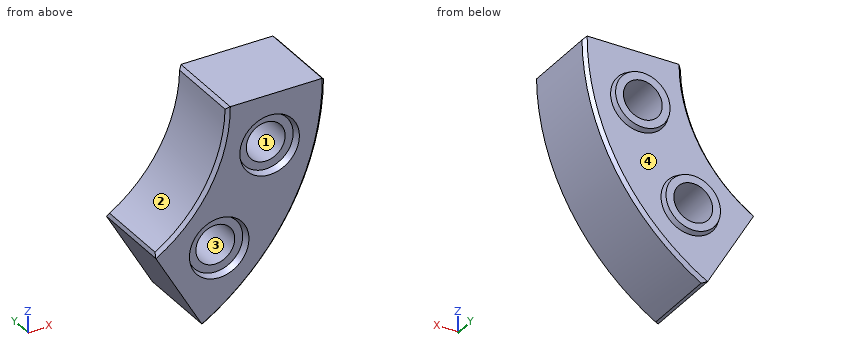
```python
from build123d import *
from OCP.BRepFilletAPI import BRepFilletAPI_MakeChamfer

# Parameters (mm, degrees)
SKETCH1_R           = 30
BOSS_EXTRUDE1_DEPTH = 127
BOSS_EXTRUDE2_START = 8
SKETCH2_R           = 45
SKETCH2_R_2         = 30
BOSS_EXTRUDE2_DEPTH = 8
CHAMFER1_SIZE       = 2.911761874
CHAMFER1_SIZE_2     = 8
CUT_EXTRUDE1_START  = -10
SKETCH3_R           = 46
SKETCH3_R_2         = 30
CUT_EXTRUDE1_DEPTH  = 10
CHAMFER2_SIZE       = 3.639702343
CHAMFER2_SIZE_2     = 10


# Some blends are built 0.0001 mm under size
with BuildPart() as part:
    # Sketch1 → Boss-Extrude1 (new body)
    with BuildSketch(Plane(origin=(0, 0, 0), x_dir=(1, 0, 0), z_dir=(0, 1, 0))):
        with BuildLine():
            Line((225, 0), (377, 0))
            ThreePointArc((377, 0), (326.491577227, 188.5), (188.5, 326.491577227))
            Line((188.5, 326.491577227), (112.5, 194.855715852))
            ThreePointArc((112.5, 194.855715852), (194.855715851, 112.5), (225, 0))
        make_face()
        with Locations(Location((212.839141137, 212.839141137, 0), (0, 0, 270))):
            Circle(SKETCH1_R, mode=Mode.SUBTRACT)
        with Locations(Location((290.743673713, 77.904532576, 0), (0, 0, 270))):
            Circle(SKETCH1_R, mode=Mode.SUBTRACT)
    extrude(amount=-BOSS_EXTRUDE1_DEPTH)

    # Sketch2 → Boss-Extrude2 (add)
    # profile 1 of 2: a face of its own
    with BuildSketch(Plane(origin=(0, 0, 0), x_dir=(1, 0, 0), z_dir=(0, 1, 0)).offset(BOSS_EXTRUDE2_START)):
        with Locations(Location((212.839141137, 212.839141137, 0), (0, 0, 270))):
            Circle(SKETCH2_R)
        with Locations(Location((212.839141137, 212.839141137, 0), (0, 0, 270))):
            Circle(SKETCH2_R_2, mode=Mode.SUBTRACT)
    # profile 2 of 2: a face of its own
    with BuildSketch(Plane(origin=(0, 0, 0), x_dir=(1, 0, 0), z_dir=(0, 1, 0)).offset(BOSS_EXTRUDE2_START)):
        with Locations(Location((290.743673713, 77.904532576, 0), (0, 0, 270))):
            Circle(SKETCH2_R)
        with Locations(Location((290.743673713, 77.904532576, 0), (0, 0, 270))):
            Circle(SKETCH2_R_2, mode=Mode.SUBTRACT)
    extrude(amount=-BOSS_EXTRUDE2_DEPTH)

    # Chamfer1
    chamfer1_edges_1 = [part.edges().sort_by_distance(p)[0] for p in [
        (212.839141137, 8, -257.839141137),
    ]]
    chamfer1_side_1 = [part.faces().sort_by_distance(p)[0] for p in [
        (212.839141137, 8, -257.7809059),
    ]]
    chamfer1_edges_2 = [part.edges().sort_by_distance(p)[0] for p in [
        (290.743673713, 8, -122.904532576),
    ]]
    chamfer1_side_2 = [part.faces().sort_by_distance(p)[0] for p in [
        (290.743673713, 8, -122.846297338),
    ]]
    chamfer1 = BRepFilletAPI_MakeChamfer(part.part.solid().wrapped)
    for e in chamfer1_edges_1:
        chamfer1.Add(CHAMFER1_SIZE - 0.0001, CHAMFER1_SIZE_2 - 0.0001, e.wrapped, chamfer1_side_1[0].wrapped)
    for e in chamfer1_edges_2:
        chamfer1.Add(CHAMFER1_SIZE - 0.0001, CHAMFER1_SIZE_2 - 0.0001, e.wrapped, chamfer1_side_2[0].wrapped)
    add(Compound.cast(chamfer1.Shape()), mode=Mode.REPLACE)  # a hair under: the kernel refuses the full size

    # Sketch3 → Cut-Extrude1 (cut)
    # profile 1 of 2: a face of its own
    with BuildSketch(Plane.XZ.offset(127).offset(CUT_EXTRUDE1_START)):
        with Locations(Location((290.743673713, -77.904532576, 0), (0, 0, 270))):
            Circle(SKETCH3_R)
        with Locations(Location((290.743673713, -77.904532576, 0), (0, 0, 90))):
            Circle(SKETCH3_R_2, mode=Mode.SUBTRACT)
    # profile 2 of 2: a face of its own
    with BuildSketch(Plane.XZ.offset(127).offset(CUT_EXTRUDE1_START)):
        with Locations(Location((212.839141137, -212.839141137, 0), (0, 0, 270))):
            Circle(SKETCH3_R)
        with Locations(Location((212.839141137, -212.839141137, 0), (0, 0, 90))):
            Circle(SKETCH3_R_2, mode=Mode.SUBTRACT)
    extrude(amount=CUT_EXTRUDE1_DEPTH, mode=Mode.SUBTRACT)

    # Chamfer2
    chamfer2_edges_1 = [part.edges().sort_by_distance(p)[0] for p in [
        (290.743673713, -117, -31.904532576),
    ]]
    chamfer2_side_1 = [part.faces().sort_by_distance(p)[0] for p in [
        (290.743673713, -117, -31.977326623),
    ]]
    chamfer2_edges_2 = [part.edges().sort_by_distance(p)[0] for p in [
        (212.839141137, -117, -166.839141137),
    ]]
    chamfer2_side_2 = [part.faces().sort_by_distance(p)[0] for p in [
        (212.839141137, -117.072794047, -166.839141137),
    ]]
    chamfer2 = BRepFilletAPI_MakeChamfer(part.part.solid().wrapped)
    for e in chamfer2_edges_1:
        chamfer2.Add(CHAMFER2_SIZE - 0.0001, CHAMFER2_SIZE_2 - 0.0001, e.wrapped, chamfer2_side_1[0].wrapped)
    for e in chamfer2_edges_2:
        chamfer2.Add(CHAMFER2_SIZE_2 - 0.0001, CHAMFER2_SIZE - 0.0001, e.wrapped, chamfer2_side_2[0].wrapped)
    add(Compound.cast(chamfer2.Shape()), mode=Mode.REPLACE)  # a hair under: the kernel refuses the full size

    # Chamfer3
    # the kernel refuses this chamfer: 5 mm, written as the material it takes off along each edge
    with BuildSketch(Plane(origin=(0, -127, 0), x_dir=(0.9994181981512107, 0, 0.03410667389511293), z_dir=(-0.03410667389511293, 0, 0.9994181981512107))) as chamfer3_piece_1:
        with BuildLine():
            Line((371.858578644, -0.141421356), (377.141421356, 5.141421356))
            Line((377.141421356, 5.141421356), (377.241421356, 5.141421356))
            ThreePointArc((377.241421356, 5.141421356), (377.1, 2.570710678), (377.1, 0))
            Line((377.1, 0), (377, -0.1))
            ThreePointArc((377, -0.1), (374.429289322, -0.1), (371.858578644, -0.241421356))
            Line((371.858578644, -0.241421356), (371.858578644, -0.141421356))
        make_face()
    revolve(axis=Axis((0, -127, 0), (0, 1, 0)), revolution_arc=63.90909507, mode=Mode.SUBTRACT)
    with BuildSketch(Plane(origin=(0, -127, 0), x_dir=(0.4497094956032867, 0, -0.8931748818480272), z_dir=(-0.8931748818480272, 0, -0.4497094956032867))) as chamfer3_piece_2:
        with BuildLine():
            Line((230.141421356, 0.141421356), (224.858578644, -5.141421356))
            Line((224.858578644, -5.141421356), (224.758578644, -5.141421356))
            ThreePointArc((224.758578644, -5.141421356), (224.9, -2.570710678), (224.9, 0))
            Line((224.9, 0), (225, 0.1))
            ThreePointArc((225, 0.1), (227.570710678, 0.1), (230.141421356, 0.241421356))
            Line((230.141421356, 0.241421356), (230.141421356, 0.141421356))
        make_face()
    revolve(axis=Axis((0, -127, 0), (0, -1, 0)), revolution_arc=66.549905963, mode=Mode.SUBTRACT)
    with BuildSketch(Plane(origin=(0, 0, 0), x_dir=(0.9994181981512107, 0, 0.03410667389511288), z_dir=(-0.03410667389511288, 0, 0.9994181981512107))) as chamfer3_piece_3:
        with BuildLine():
            Line((377.141421356, -5.141421356), (371.858578644, 0.141421356))
            Line((371.858578644, 0.141421356), (371.858578644, 0.241421356))
            ThreePointArc((371.858578644, 0.241421356), (374.429289322, 0.1), (377, 0.1))
            Line((377, 0.1), (377.1, 0))
            ThreePointArc((377.1, 0), (377.1, -2.570710678), (377.241421356, -5.141421356))
            Line((377.241421356, -5.141421356), (377.141421356, -5.141421356))
        make_face()
    revolve(axis=Axis((0, 0, 0), (0, 1, 0)), revolution_arc=63.90909507, mode=Mode.SUBTRACT)
    with BuildSketch(Plane(origin=(0, 0, 0), x_dir=(0.4497094956032867, 0, -0.8931748818480272), z_dir=(-0.8931748818480272, 0, -0.4497094956032867))) as chamfer3_piece_4:
        with BuildLine():
            Line((224.858578644, 5.141421356), (230.141421356, -0.141421356))
            Line((230.141421356, -0.141421356), (230.141421356, -0.241421356))
            ThreePointArc((230.141421356, -0.241421356), (227.570710678, -0.1), (225, -0.1))
            Line((225, -0.1), (224.9, 0))
            ThreePointArc((224.9, 0), (224.9, 2.570710678), (224.758578644, 5.141421356))
            Line((224.758578644, 5.141421356), (224.858578644, 5.141421356))
        make_face()
    revolve(axis=Axis((0, 0, 0), (0, -1, 0)), revolution_arc=66.549905963, mode=Mode.SUBTRACT)
    with BuildSketch(Plane(origin=(112.5, 12.726295315, -194.855715852), x_dir=(0.4760148236193062, 0, -0.8794372562580466), z_dir=(0, -1, 0))) as chamfer3_piece_5:
        with BuildLine():
            Line((5.090518126, 0), (-0.33429411, 5.023891374))
            Line((-0.33429411, 5.023891374), (-0.434172994, 5.018971161))
            ThreePointArc((-0.434172994, 5.018971161), (-0.183141977, 2.511326919), (-0.099962242, -0.00274777))
            Line((-0.099962242, -0.00274777), (0.00274777, -0.099962242))
            ThreePointArc((0.00274777, -0.099962242), (2.546085101, -0.030050788), (5.093265896, -0.099962242))
            Line((5.093265896, -0.099962242), (5.090518126, 0))
        make_face()
    extrude(amount=152.452590629, mode=Mode.SUBTRACT)
    with BuildSketch(Plane(origin=(188.5, 13.026648977, -326.491577227), x_dir=(-0.5236311743551006, 0, 0.8519450646863905), z_dir=(0, -1, 0))) as chamfer3_piece_6:
        with BuildLine():
            Line((5.176029718, 0), (-0.249663351, -5.204674974))
            Line((-0.249663351, -5.204674974), (-0.349653457, -5.203268263))
            ThreePointArc((-0.349653457, -5.203268263), (-0.162620276, -2.601558906), (-0.099962166, 0.002750537))
            Line((-0.099962166, 0.002750537), (0.002750537, 0.099962166))
            ThreePointArc((0.002750537, 0.099962166), (2.588807445, 0.0288048), (5.178780254, 0.099962166))
            Line((5.178780254, 0.099962166), (5.176029718, 0))
        make_face()
    extrude(amount=153.053297954, mode=Mode.SUBTRACT)
    with BuildSketch(Plane(origin=(377, 13.026648977, 0), x_dir=(0.02042205911014994, 0, -0.9997914480038833), z_dir=(0, -1, 0))) as chamfer3_piece_7:
        with BuildLine():
            Line((5.210659591, 0), (-0.248004097, -5.170084874))
            Line((-0.248004097, -5.170084874), (-0.347983242, -5.168042668))
            ThreePointArc((-0.347983242, -5.168042668), (-0.152811741, -2.584453961), (-0.099979145, 0.002042206))
            Line((-0.099979145, 0.002042206), (0.002042206, 0.099979145))
            ThreePointArc((0.002042206, 0.099979145), (2.60636271, 0.037782504), (5.214045418, 0.099942664))
            Line((5.214045418, 0.099942664), (5.210659591, 0))
        make_face()
    extrude(amount=153.053297954, mode=Mode.SUBTRACT)
    with BuildSketch(Plane(origin=(225, 12.726295315, 0), x_dir=(-0.03895191023079492, 0, -0.999241086369737), z_dir=(0, -1, 0))) as chamfer3_piece_8:
        with BuildLine():
            Line((5.0350012, 0), (-0.337980103, 5.0792858))
            Line((-0.337980103, 5.0792858), (-0.437904212, 5.075390609))
            ThreePointArc((-0.437904212, 5.075390609), (-0.199029377, 2.538471922), (-0.099924109, -0.003895191))
            Line((-0.099924109, -0.003895191), (0.003895191, -0.099924109))
            ThreePointArc((0.003895191, -0.099924109), (2.517945165, -0.016000711), (5.036723207, -0.099985172))
            Line((5.036723207, -0.099985172), (5.0350012, 0))
        make_face()
    extrude(amount=152.452590629, mode=Mode.SUBTRACT)


solid = part.part
```
Work out the finished part from the listing and answer in its coordinate system (mm). Face numbers are marked on the shaded views. Coordinates: 2 decimals unless noted, no trailing zeros. Write each loop counter-clockwise with the first axis right and the second up, starting at its lowest first coordinate (ties: lowest second). Pieces come first, ordered by that corner, then holes.
Q1. A cutting plane is placed at A-A, the plane y = -12.5. Give the vertices of the cut face in (x, z), then the cut area to 3 significant figures.
Q2. Each of these flat-tipped pins is pushed along its axis until it touches: pin 1 Ø4 at (y, z) = (-24.5, -176.5) entering from -X; pin 2 Ø5 at (x, y) = (321.5, -93.5) entering from -Z; pin 3 Ø6 at (x, y) = (349.5, -42) entering from -Z. Where does it stop, or does it pass through?
Q3. Find the intervals of material crossed by line 1 (Z direction, x = 235, y = -85.5); line 2 (Z direction, x = 265.5, y = -61); line 3 (X direction, y = -49, z = -235), in increasing order.
Q4. Determine the mould class of the marked faces 1, 2, 3 and 4 for opening direction X: released by +X, released by -X, zero draft, split by the parting line, or undercut.
Findings below:
1. outline: (114.97, -199.14) - (185.98, -322.13) - (192.87, -323.93) arc R377 ccw to (376.97, -5.07) - (371.97, 0) - (229.95, 0) - (224.95, -4.89) arc R225 cw to (116.71, -192.36) - close; hole circle Ø60 at (212.84, -212.84); hole circle Ø60 at (290.74, -77.9)
1. area: 42,200 mm2
2. pin 1: stops at x = 136.98
2. pin 2: stops at z = -200.92
2. pin 3: stops at z = -148.55
3. line 1: z = -294.79 to -233.06, -192.62 to 0
3. line 2: z = -267.65 to -94.11, -61.69 to 0
3. line 3: x = 135.68 to 192.62, 233.06 to 294.79
4. face 1: undercut
4. face 2: released by -X
4. face 3: undercut
4. face 4: zero draft
